from build123d import *

# Parameters (mm, degrees)
BOSS_EXTRUDE1_DEPTH   = 28.575
CHAMFER1_SIZE         = 4.7625
FILLET1_R             = 3.175
FILLET2_R             = 1.5875
F_8_CLEARANCE_HOLE1_D = 3.81


with BuildPart() as part:
    # Sketch1 → Boss-Extrude1 (new body)
    with BuildSketch(Plane(origin=(0, 0, 0), x_dir=(0, 0, -1), z_dir=(1, 0, 0))):
        with BuildLine():
            Line((0, 0), (0, 50.8))
            Line((0, 50.8), (14.399754562, 50.8))
            ThreePointArc((14.399754562, 50.8), (2.654588994, 25.4), (14.399754562, 0))
            Line((14.399754562, 0), (0, 0))
        make_face()
    extrude(amount=BOSS_EXTRUDE1_DEPTH)

    # Chamfer1
    chamfer1_edges = [part.edges().sort_by_distance(p)[0] for p in [
        (14.2875, 0, 0),
    ]]
    chamfer(chamfer1_edges, length=CHAMFER1_SIZE)

    # Fillet1
    fillet1_edges = [part.edges().sort_by_distance(p)[0] for p in [
        (14.2875, 0, -4.7625),
        (14.2875, 4.7625, 0),
        (14.2875, 50.8, 0),
    ]]
    fillet(fillet1_edges, radius=FILLET1_R)

    # Fillet2
    fillet2_edges = [part.edges().sort_by_distance(p)[0] for p in [
        (14.2875, 50.8, -14.399754562),
        (14.2875, 0, -14.399754562),
    ]]
    fillet(fillet2_edges, radius=FILLET2_R)

    # #8 Clearance Hole1 (through all)
    with Locations(Plane(origin=(28.575, 0, 0), x_dir=(0, 0, -1), z_dir=(1, 0, 0))):
        with Locations((4.445, 46.355), (4.445, 6.603679285)):
            Hole(F_8_CLEARANCE_HOLE1_D / 2)


solid = part.part
For this review, take the finished solid that the model builds, in its own axes (mm). Give positions to 0.01 mm unless a question says otherwise; leave off trailing zeros. Loops run counter-clockwise (first coordinate to the right, second up) from the corner with the lowest first, then second, coordinate; pieces in that order, holes last.
Item 1: Take a section at C-C, the plane x = 26.75. Give the number of separate pieces and of enclosed holes in the cut face, and give its area (3 significant figures).
Item 2: Insertion check: pin 1 (1 mm diameter, centred on y = 40.5, z = -7.5, fed in from -X); pin 2 (1 mm diameter, centred on x = 9, z = -2, fed in from +Y). Each pin has a flat end and moves straight along its axis. Give the tip position at first contact, or say it passes through.
Item 3: Take a section at A-A, the plane y = 8. State the section outline as (x, z) points (3 decimals), and give its area (3 significant figures).
Item 4: Take a section at B-B, the plane z = -7.25. State the section outline as (x, y) points (3 decimals).
Item 5: For line 1 along Y through (x, z) = (25.5, -5.5); line 2 along Y through (x, z) = (10, -11); line 3 along Y through (x, z) = (15, -10), list the stretches that pass through material, from the lowest coordinate up.
Item 6: Take a section at D-D, the plane y = 38. State the section outline as (x, z) points (3 decimals), and give its area (3 significant figures).
Item 7: Draft analysis for pull direction Z (two halves, no side actions). For faces 1 (the flat face through (14, 0, -8)), 2 (the cylindrical face through (14.087, 44.665, -3.566)), 3 (the cylindrical face through (14.49, 49.85, -0.91)), 4 (the cylindrical face through (14.49, 0.98, -11.91)), state which applies: +Z half, -Z half, draft (parallel to the pull), parting line (faces both ways), or undercut.
Calculated:
1. separate pieces: 1
1. enclosed holes: 2
1. area: 274 mm2
2. pin 1: passes through
2. pin 2: stops at y = 50.73
3. outline: (0, -7.556) - (28.575, -7.556) - (28.575, -5.741) - (0, -5.741) - close; (0, -3.149) - (28.575, -3.149) - (28.575, 0) - (0, 0) - close
3. area: 142 mm2
4. outline: (0, 0) - (28.575, 0) - (28.575, 8.51) - (0, 8.51) - close; (0, 42.29) - (28.575, 42.29) - (28.575, 50.8) - (0, 50.8) - close
5. line 1: y = 0.05 to 5.02, 8.19 to 11.92, 38.88 to 44.77, 47.94 to 50.8
5. line 2: y = 0.1 to 3.34, 47.46 to 50.7
5. line 3: y = 0 to 4.52, 46.28 to 50.8
6. outline: (0, -5.127) - (28.575, -5.127) - (28.575, 0) - (0, 0) - close
6. area: 147 mm2
7. face 1: draft
7. face 2: undercut
7. face 3: +Z half
7. face 4: -Z half
